Could you check a few things on this model? Use its own coordinates, in mm. Face numbers are marked on the shaded views. A direction names the side the tool comes from. Coordinates: 2 decimals unless noted, no trailing zeros. Loops run counter-clockwise (first coordinate to the right, second up) from the corner with the lowest first, then second, coordinate; pieces in that order, holes last. Notation, with made-up numbers: (23, 68) -> (30, 68) arc R26 cw to (30, 107) -> close; hole circle Ø9 at (2, 28.5). An arc over 180 degrees is marked (long way). One line per question, with ' | ' between items.
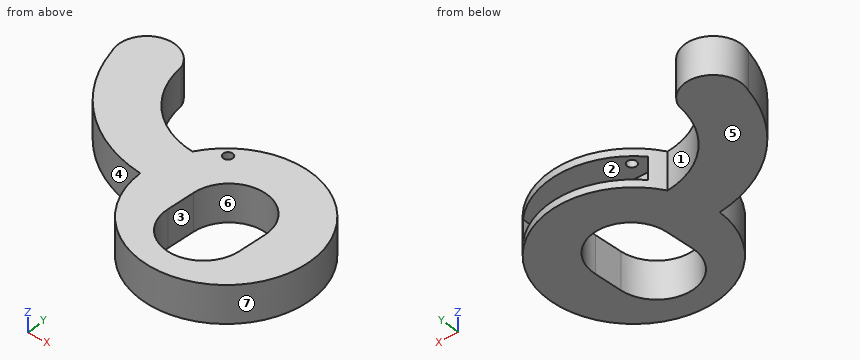
Autodesk Inventor part; units mm, degrees
ref_plane "Plano de trabalho1" through (0, 4.5, 0) normal (0, 1, 0) x (-1, 0, 0)
ref_plane "YZ Plane" through (0, 0, 0) normal (1, 0, 0) x (0, 1, 0)
ref_plane "XY Plane" through (0, 0, 0) normal (0, 0, 1) x (1, 0, 0)
sketch "Esboço1" plane through (0, 0, 0) normal (0, 0, 1) x (1, 0, 0)
  circle A0 centre (0, 0) radius 4.5
  dimension "d0" = 9
extrude "Extrusão1" add sketch "Esboço1" along normal blind 2
sketch "Esboço2" plane through (0, 0, 2) normal (0, 0, 1) x (1, 0, 0)
  circle A0 centre (0, 0) radius 4.5
  arc A1 (-10.4751, 5.4783) -> (-4.5, 0.0043) centre (-3.6315, 6.9502) ccw
  arc A2 (-7.6364, 6.4456) -> (-10.4751, 5.4783) centre (-9.0687, 6) ccw
  arc A3 (-7.6364, 6.4456) -> (-3.7747, 2.4498) centre (-3.3457, 6.7283) ccw
  dimension "d3" = 7
  dimension "d4" = 4.3
  dimension "d5" = 1.5
  dimension "d6" = 6
extrude "Extrusão2" add sketch "Esboço2" against normal blind 2 contours A0 A1 A2 A3
sketch "Esboço4" plane through (0, 0, 2) normal (0, 0, 1) x (1, 0, 0)
  line L0 (-0.335, -0.9422) -> (0.1675, 0.4711) construction
  line L1 (-2.0175, 0.3756) -> (-2.1372, -1.1196)
  line L2 (1.85, -1.439) -> (1.9698, 0.0562)
  arc A0 (1.9698, 0.0562) -> (-2.0175, 0.3756) centre (-0.0239, 0.2159) ccw
  arc A1 (-2.1372, -1.1196) -> (1.85, -1.439) centre (-0.1436, -1.2793) ccw
  point P0 (-0.0837, -0.2356)
  dimension "d11" = 1.5
  dimension "d12" = 4
extrude "Extrusão3" cut sketch "Esboço4" against normal blind 2
ref_plane "Plano de trabalho1" through (0, 4.5, 0) normal (0, 1, 0) x (-1, 0, 0)
sketch "Esboço5" plane through (0, 4.5, 0) normal (0, 1, 0) x (-1, 0, 0)
  line L0 (-3.25, 1.6) -> (3.2747, 1.6)
  line L1 (3.2747, 1.6) -> (3.2747, 0.4)
  line L2 (3.2747, 0.4) -> (-3.25, 0.4)
  line L3 (-3.25, 0.4) -> (-3.25, 1.6)
  line L4 (-3.25, 1.6) -> (3.2747, 0.4) construction
  line L5 (3.2747, 1.6) -> (-3.25, 0.4) construction
  line L6 (4.5, 0) -> (-4.5, 0)
  line L7 (4.5, 2) -> (-4.5, 2)
  line L8 (3.7747, 0) -> (3.7747, 2)
  line L9 (-4.5, 2) -> (-4.5, 0)
  line L10 (-4.5, 0) -> (-4.5, 2)
  point P0 (0, 0)
  point P1 (0.0124, 1)
  dimension "d16" = 0.4
  dimension "d17" = 0.4
  dimension "d18" = 0.5
  dimension "d19" = 1.25
extrude "Extrusão4" cut sketch "Esboço5" against normal blind 2.2 contours L0 L1 L2 L3
sketch "Esboço6" plane through (0, 0, 2) normal (0, 0, 1) x (1, 0, 0)
  circle A0 centre (-2.473, 3.141) radius 0.25
  line L0 (0, -6.9) -> (0, 9.9)
  line L1 (-13.5824, 0) -> (7.5137, 0)
  point P0 (0, 0)
  dimension "d22" = 0.5
  dimension "d28" = 2.473
  dimension "d29" = 3.141
extrude "Extrusão5" cut sketch "Esboço6" against normal blind 0.5
sketch "Esboço8" plane through (0, 2.3, 0) normal (0, 1, 0) x (1, 0, 0)
  line L0 (1.9698, -2) -> (1.9698, 0)
  circle A0 centre (1.9698, -1) radius 0.25
  point P0 (0, 0)
  dimension "d30" = 0.5
extrude "Extrusão7" cut sketch "Esboço8" against normal blind 0.1
properties material "Liga de Nickel-Copper 400"
1) On a 3-axis mill with a long thin cutter (end or side, diameter ignored), from which of +Z, -Z, +X, -X, +Y, -Y can I reach the whole of each face in a straight line? I mean the marked faces 1, 2, 3 and 4. Say none if no direction works.
Data:
face 1: +Z, -Z, +Y | face 2: +Y | face 3: +Z, -Z | face 4: +Z, -Z, -X, -Y
2) We'd pull the mould along Y, two halves only. Please class the marked faces 5, 6 and 7: pulls with the +Y half, pulls with the -Y half, needs draft (parallel to the pull), parting line crosses it, or undercut.
Data:
face 5: needs draft | face 6: undercut | face 7: parting line crosses it
3) If we section it at A-A on z = 1: Please give me the cut outline in (x, y).
Data:
outline: (-10.48, 5.48) arc R7 ccw to (-4.5, 0) arc R4.5 ccw (long way) to (3.25, 3.11) -> (3.25, 2.3) -> (2.22, 2.3) -> (2.22, 2.2) -> (1.72, 2.2) -> (1.72, 2.3) -> (-3.27, 2.3) -> (-3.27, 3.09) arc R4.5 ccw to (-3.77, 2.45) arc R4.3 cw to (-7.64, 6.45) arc R1.5 ccw (long way) to start; hole (-2.14, -1.12) arc R2 ccw to (1.85, -1.44) -> (1.97, 0.06) arc R2 ccw to (-2.02, 0.38) -> close
4) I'm going to push flat-ended pins straight in: pin 1 Ø1 at (x, z) = (-4.5, 1) entering from +Y; pin 2 Ø1 at (x, z) = (1, 1) entering from +Y. Where does each tip first touch, or does it pass through?
Data:
pin 1: y = 2.76 | pin 2: y = 2.3
5) If we section it at C-C on y = -3: Please give me the cut outline in (x, z).
Data:
outline: (-3.35, 0) -> (-1.16, 0) -> (-1.16, 2) -> (-3.35, 2) -> close; (0.88, 0) -> (3.35, 0) -> (3.35, 2) -> (0.88, 2) -> close
6) If we section it at B-B on x = 0: Please give me the cut outline in (y, z).
Data:
outline: (-4.5, 0) -> (-3.27, 0) -> (-3.27, 2) -> (-4.5, 2) -> close; (2.22, 0) -> (4.5, 0) -> (4.5, 0.4) -> (2.3, 0.4) -> (2.3, 1.6) -> (4.5, 1.6) -> (4.5, 2) -> (2.22, 2) -> close
7) I need wall thicknesses on line 1 along X through (y, z) = (2.75, 1.4); line 2 along X through (y, z) = (-0.5, 1.6); line 3 along X through (y, z) = (-1, 1.35). Which ranges of each line are inside material? Lowest first, please. Write a range as from..to.
Data:
line 1: -9.23..-4.98, -3.56..-3.27, 3.25..3.56 | line 2: -4.47..-2.09, 1.93..4.47 | line 3: -4.39..-2.13, 1.89..4.39
8) If we section it at D-D on y = 4.25: Please give me the cut outline in (x, z), and give its area (3 significant figures).
Data:
outline: (-10.09, 0) -> (-6.86, 0) -> (-6.86, 2) -> (-10.09, 2) -> close; (-1.48, 0) -> (1.48, 0) -> (1.48, 0.4) -> (-1.48, 0.4) -> close; (-1.48, 1.6) -> (1.48, 1.6) -> (1.48, 2) -> (-1.48, 2) -> close | area: 8.83 mm²
